Verification items for the finished model (mm, model axes). Face numbers are marked on the shaded views. Coordinates: 2 decimals unless noted, no trailing zeros. Write each loop counter-clockwise with the first axis right and the second up, starting at its lowest first coordinate (ties: lowest second). Pieces come first, ordered by that corner, then holes. Notation, with made-up numbers: (11.25, 2) -> (40.25, 2) arc R35 cw to (40.25, 34) -> close; hole circle Ø3 at (69, 70). An arc over 180 degrees is marked (long way). Write each question's results on one line, items separated by ' | '. Start each with the question number.
Autodesk Inventor part; units mm, degrees
ref_plane "YZ Plane" through (0, 0, 0) normal (1, 0, 0) x (0, 1, 0)
ref_plane "XZ Plane" through (0, 0, 0) normal (0, 1, 0) x (-1, 0, 0)
ref_plane "XY Plane" through (0, 0, 0) normal (0, 0, 1) x (1, 0, 0)
sketch "Sketch1" plane through (0, 0, 0) normal (0, 1, 0) x (-1, 0, 0)
  line L0 (0, 0) -> (-1.5, 0)
  line L1 (-1.5, 0) -> (-1.5, 41)
  line L2 (-1.5, 41) -> (0, 41) construction
  line L3 (0, 41) -> (0, 0)
  line L4 (0, 0) -> (-27, 0)
  line L5 (-27, 0) -> (-27, 1.5)
  line L6 (-27, 1.5) -> (0, 1.5)
  line L7 (0, 1.5) -> (0, 0)
  line L8 (-27, 1.5) -> (-25.5, 1.5)
  line L9 (-25.5, 1.5) -> (-25.5, -3)
  line L10 (-25.5, -3) -> (-27, -3)
  line L11 (-27, -3) -> (-27, 1.5)
  arc A0 (-2.25, 42.5) -> (0.75, 42.5) centre (-0.75, 42.5) ccw
  line L12 (-0.75, 41) -> (-0.75, 42.5) construction
  line L13 (-0.75, 42.5) -> (0.75, 42.5) construction
  arc A1 (1.75, 42.5) -> (0.75, 42.5) centre (1.25, 42.5) ccw
  arc A2 (-3.25, 42.5) -> (1.75, 42.5) centre (-0.75, 42.5) ccw
  arc A3 (-2.25, 42.5) -> (-3.25, 42.5) centre (-2.75, 42.5) ccw
  point P0 (-0.75, 41)
  point P1 (-25.5, 0)
  point P2 (0, 40.1152)
  point P3 (-1.5, 40.1152)
  point P4 (-1.5, 1.5)
  dimension "d0" = 1.5
  dimension "d1" = 41
  dimension "d2" = 27
  dimension "d3" = 1.5
  dimension "d4" = 1.5
  dimension "d5" = 4.5
  dimension "d6" = 3
  dimension "d7" = 1
extrude "Extrusion1" add sketch "Sketch1" along normal blind 163.5125
fillet "Fillet1" radius 2.5 2 edges at (0, 81.7562, 0) (27, 81.7562, 1.5)
fillet "Fillet2" radius 1 2 edges at (1.5, 81.7562, 1.5) (25.5, 81.7562, 0)
fillet "Fillet3" radius 0.5 4 edges at (0, 81.7562, 40.1152) (1.5, 81.7562, 40.1152) (27, 81.7562, -3) (25.5, 81.7562, -3)
properties part number "Light Cover"
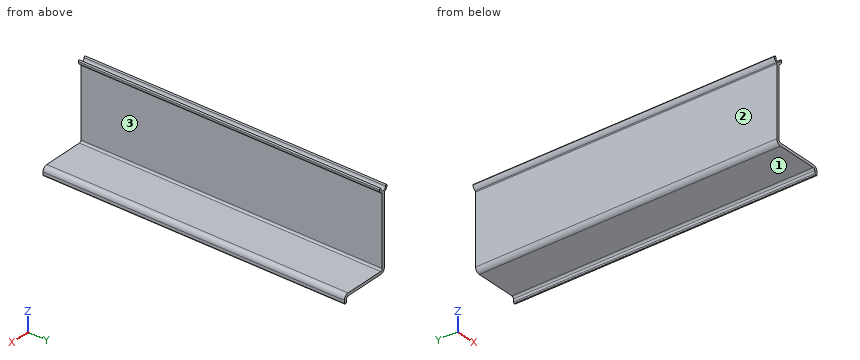
1. Mould release check, pull along Z, two halves, no side actions. Record for the marked faces 1, 2 and 3: +Z half, -Z half, draft (parallel to the pull), parting line (faces both ways), or undercut.
2. Sectioned sample at A-A on y = 74.5. Record the cut outline in (x, z).
3. Sectioned sample at C-C on z = 19. Record the cut outline in (x, y).
4. Sectioned sample at B-B on x = 15.5. Record the cut outline in (y, z), plus the area to 3 significant figures.
5. Material ranges on probe 1 along X at (y, z) = (132, 20); probe 2 along Z at (x, y) = (25, 155.5), recorded low to high. Write a range as from..to.
6. Depth check by flat-ended pin: pin 1 Ø4 at (x, y) = (18, 16.5) entering from -Z; pin 2 Ø8 at (x, z) = (8.5, 25.5) entering from +Y; pin 3 Ø0.8 at (y, z) = (97, -1.5) entering from -X; pin 4 Ø2 at (y, z) = (91, 14) entering from +X. Enter the tip coordinate at first touch or a pass-through.
Computed values:
1) face 1: -Z half | face 2: draft | face 3: undercut
2) outline: (-1.75, 42.5) arc R2.5 ccw to (-0.29, 40.23) arc R0.5 cw to (0, 39.77) -> (0, 2.5) arc R2.5 ccw to (2.5, 0) -> (24.5, 0) arc R1 cw to (25.5, -1) -> (25.5, -2.5) arc R0.5 ccw to (26, -3) -> (26.5, -3) arc R0.5 ccw to (27, -2.5) -> (27, -1) arc R2.5 ccw to (24.5, 1.5) -> (2.5, 1.5) arc R1 cw to (1.5, 2.5) -> (1.5, 39.77) arc R0.5 cw to (1.79, 40.23) arc R2.5 ccw to (3.25, 42.5) arc R0.5 ccw to (2.25, 42.5) arc R1.5 cw to (-0.75, 42.5) arc R0.5 ccw to start
3) outline: (0, 0) -> (1.5, 0) -> (1.5, 163.51) -> (0, 163.51) -> close
4) outline: (0, 0) -> (163.51, 0) -> (163.51, 1.5) -> (0, 1.5) -> close | area: 245 mm^2
5) probe 1: x = 0..1.5 | probe 2: z = -0.13..1.45
6) pin 1: stops at z = 0 | pin 2: passes through | pin 3: stops at x = 25.5 | pin 4: stops at x = 1.5
